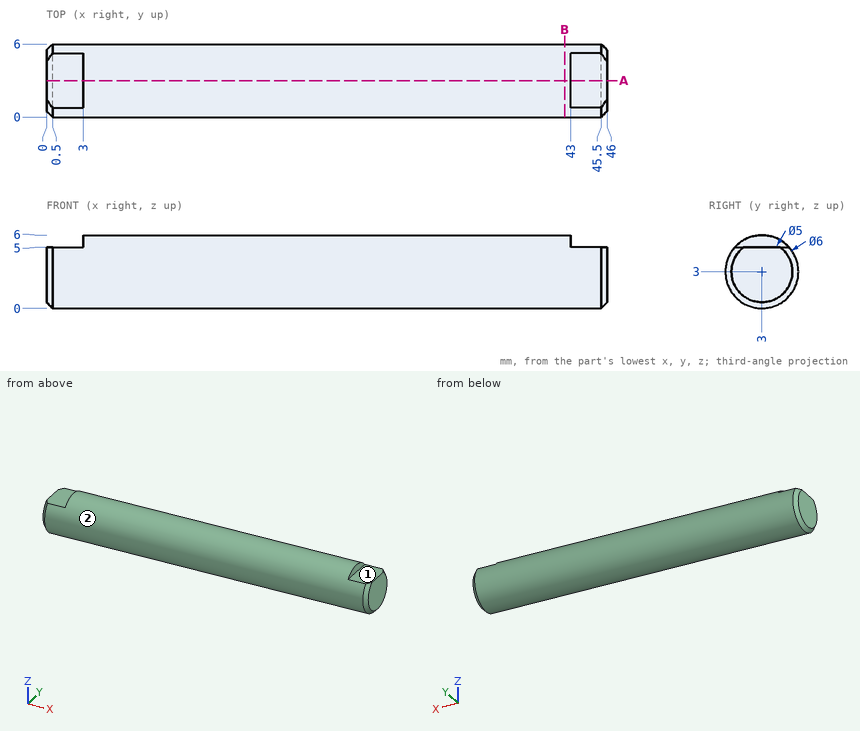
Here's the drawing with two shaded views (mm, measured from the low corner). I have some questions. A direction names the side the tool comes from. Coordinates: 2 decimals unless noted, no trailing zeros. Write each loop counter-clockwise with the first axis right and the second up, starting at its lowest first coordinate (ties: lowest second). Pieces come first, ordered by that corner, then holes. Notation, with made-up numbers: (-1.5, 84.25) -> (28.5, 84.25) arc R16 cw to (28.5, 96.25) -> close; hole circle Ø3 at (-22, 2). An arc over 180 degrees is marked (long way). Use a Markdown table: item, result. Add a question column.
(1) Please list where these lines run through material, in increasing order: line 1 (Z direction, x = 27.5, y = 1); line 2 (Z direction, x = 6, y = 0.5); line 3 (Y direction, x = 40.5, z = 2.3).
(2) I'm going to push flat-ended pins straight in: P1, Ø2, axis at x = 14, y = 4.5, coming from the -Z side; P2, Ø0.8, axis at y = 2, z = 5.5, coming from the +X side; P3, Ø1.5, axis at x = 2, y = 3.5, coming from the +Z side. Where does each tip first touch, or does it pass through?
(3) For the marked faces 1 and 2, which set-ups out of +Z, -Z, +X, -X, +Y, -Y let a thin tool reach every point of the face, with its end or its side?
(4) If we section it at B-B, the plane x = 42.5: Write out the boundary of the cut face in (y, z), and give its area (3 significant figures).
(5) If we section it at A-A, the plane y = 3: Write out the boundary of the cut face in (x, z), and give its area (3 significant figures).
Outcome:
| question | item | result |
|---|---|---|
| 1 | line 1 | z = 0.76 to 5.24 |
| 1 | line 2 | z = 1.34 to 4.66 |
| 1 | line 3 | y = 0.08 to 5.92 |
| 2 | P1 | stops at z = 0.04 |
| 2 | P2 | stops at x = 43 |
| 2 | P3 | stops at z = 5 |
| 3 | face 1 | +Z, +X, +Y, -Y |
| 3 | face 2 | +X, -X |
| 4 | outline | circle Ø6 at (3, 3) |
| 4 | area | 28.3 mm^2 |
| 5 | outline | (0, 0.5) -> (0.5, 0) -> (45.5, 0) -> (46, 0.5) -> (46, 5) -> (43, 5) -> (43, 6) -> (3, 6) -> (3, 5) -> (0, 5) -> close |
| 5 | area | 270 mm^2 |
